```python
from build123d import *

# Parameters (mm, degrees)
SKETCH1_W           = 152.4
SKETCH1_H           = 50.8
BOSS_EXTRUDE1_DEPTH = 19.05
BOSS_EXTRUDE2_DEPTH = 5.08


with BuildPart() as part:
    # Sketch1 → Boss-Extrude1 (new body)
    with BuildSketch(Plane.XY):
        Rectangle(SKETCH1_W, SKETCH1_H)
        with BuildLine():
            ThreePointArc((59.3725, 6.35), (49.2125, 16.51), (39.0525, 6.35))
            Line((39.0525, 6.35), (39.0525, -6.35))
            ThreePointArc((39.0525, -6.35), (49.2125, -16.51), (59.3725, -6.35))
            Line((59.3725, -6.35), (59.3725, 6.35))
        make_face(mode=Mode.SUBTRACT)
        with BuildLine():
            ThreePointArc((-39.0525, 6.35), (-49.2125, 16.51), (-59.3725, 6.35))
            Line((-59.3725, 6.35), (-59.3725, -6.35))
            ThreePointArc((-59.3725, -6.35), (-49.2125, -16.51), (-39.0525, -6.35))
            Line((-39.0525, -6.35), (-39.0525, 6.35))
        make_face(mode=Mode.SUBTRACT)
    extrude(amount=BOSS_EXTRUDE1_DEPTH)

    # Sketch1_3 → Boss-Extrude2 (add)
    with BuildSketch(Plane.XY):
        with BuildLine():
            Line((-39.0525, -6.35), (-39.0525, 6.35))
            ThreePointArc((-39.0525, 6.35), (-49.2125, 16.51), (-59.3725, 6.35))
            Line((-59.3725, 6.35), (-59.3725, -6.35))
            ThreePointArc((-59.3725, -6.35), (-49.2125, -16.51), (-39.0525, -6.35))
        make_face()
        with BuildLine():
            ThreePointArc((-56.007, -6.35), (-49.2125, -13.1445), (-42.418, -6.35))
            Line((-42.418, -6.35), (-42.418, 6.35))
            ThreePointArc((-42.418, 6.35), (-49.2125, 13.1445), (-56.007, 6.35))
            Line((-56.007, 6.35), (-56.007, -6.35))
        make_face(mode=Mode.SUBTRACT)
        with BuildLine():
            Line((59.3725, -6.35), (59.3725, 6.35))
            ThreePointArc((59.3725, 6.35), (49.2125, 16.51), (39.0525, 6.35))
            Line((39.0525, 6.35), (39.0525, -6.35))
            ThreePointArc((39.0525, -6.35), (49.2125, -16.51), (59.3725, -6.35))
        make_face()
        with BuildLine():
            ThreePointArc((42.418, -6.35), (49.2125, -13.1445), (56.007, -6.35))
            Line((56.007, -6.35), (56.007, 6.35))
            ThreePointArc((56.007, 6.35), (49.2125, 13.1445), (42.418, 6.35))
            Line((42.418, 6.35), (42.418, -6.35))
        make_face(mode=Mode.SUBTRACT)
    extrude(amount=BOSS_EXTRUDE2_DEPTH)


solid = part.part
```
Could you check a few things on this model? Use its own coordinates, in mm. A direction names the side the tool comes from. Coordinates: 2 decimals unless noted, no trailing zeros. Order: outer loops, then holes, each group sorted by start corner. A loop starts at its lowest first (then second) coordinate and runs counter-clockwise, first axis right, second up. Notation, with made-up numbers: M 23,29.5 L 71,29.5 A19 cw 71,42.5 Z; hole C 24.5,-40 d4. An arc over 180 degrees is marked long. Use a Markdown table: item, result. Add a question column.
Q1. I want a section at A-A on y = 2.5. List the corners of the cut face in (x, z) for me.
Q2. We'd pull the mould along Y, two halves only. Please class faces 1 (the cylindrical face through (49.063, -13.143, 2.504)), 2 (the flat face through (-1, -25.4, 9)), 3 (the cylindrical face through (-49.362, -13.143, 2.504)), 4 (the flat face through (-1, 0, 0)): pulls with the +Y half, pulls with the -Y half, needs draft (parallel to the pull), parting line crosses it, or undercut.
Q3. I'm going to push a flat-ended pin straight in: pin 1 (4 mm diameter, centred on x = 50, y = 13, fed in from +Z). Where does the tip first touch, or does it pass through?
Q4. If I drill on L1, parallel to X at y = -4.5, z = 15.5; L2, parallel to X at y = 5, z = 1; L3, parallel to Y at x = 50, z = 14.5, over which ranges is the centre line in solid material (lowest first)?
Q5. Which directions (+Z, -Z, +X, -X, +Y, -Y) give clear straight access to the entire face, cutting with the end or side of a thin tool? Please do faces 5 (the flat face through (56.007, 0, 3)), 6 (the flat face through (42, 0, 5.08)), 7 (the flat face through (-1, 0, 19.05)).
Q6. I want a section at C-C on y = 11. List the corners of the cut face in (x, z) for me, then the cut area to 3 significant figures.
Q7. I want a section at B-B on z = 7.5. List the corners of the cut face in (x, y) for me, then the cut area to 3 significant figures.
Checked values:
| question | item | result |
|---|---|---|
| 1 | outline | M -76.2,0 L -56.01,0 L -56.01,5.08 L -59.37,5.08 L -59.37,19.05 L -76.2,19.05 Z; M -42.42,0 L 42.42,0 L 42.42,5.08 L 39.05,5.08 L 39.05,19.05 L -39.05,19.05 L -39.05,5.08 L -42.42,5.08 Z; M 56.01,0 L 76.2,0 L 76.2,19.05 L 59.37,19.05 L 59.37,5.08 L 56.01,5.08 Z |
| 2 | face 1 | undercut |
| 2 | face 2 | pulls with the -Y half |
| 2 | face 3 | undercut |
| 2 | face 4 | needs draft |
| 3 | pin 1 | z = 5.08 |
| 4 | L1 | -76.2 to -59.37, -39.05 to 39.05, 59.37 to 76.2 |
| 4 | L2 | -76.2 to -56.01, -42.42 to 42.42, 56.01 to 76.2 |
| 4 | L3 | -25.4 to -16.48, 16.48 to 25.4 |
| 5 | face 5 | +Z, -Z |
| 5 | face 6 | +Z |
| 5 | face 7 | +Z, +X, -X, +Y, -Y |
| 6 | outline | M -76.2,0 L -54.17,0 L -54.17,5.08 L -58.25,5.08 L -58.25,19.05 L -76.2,19.05 Z; M -44.26,0 L 44.26,0 L 44.26,5.08 L 40.18,5.08 L 40.18,19.05 L -40.18,19.05 L -40.18,5.08 L -44.26,5.08 Z; M 54.17,0 L 76.2,0 L 76.2,19.05 L 58.25,19.05 L 58.25,5.08 L 54.17,5.08 Z |
| 6 | area | 2,300 mm² |
| 7 | outline | M -76.2,-25.4 L 76.2,-25.4 L 76.2,25.4 L -76.2,25.4 Z; hole M -59.37,-6.35 A10.16 ccw -39.05,-6.35 L -39.05,6.35 A10.16 ccw -59.37,6.35 Z; hole M 39.05,-6.35 A10.16 ccw 59.37,-6.35 L 59.37,6.35 A10.16 ccw 39.05,6.35 Z |
| 7 | area | 6,580 mm² |
